```python
from build123d import *

# Parameters (mm, degrees)
F1_DEPTH = 5
F3_DEPTH = 12
F4_R     = 1


# Not quite as in the source:
# - a feature names something its author has since deleted; it is built from what else it names


with BuildPart() as f1:
    # F0 (on Front) → F1 (new body)
    with BuildSketch(Plane.XZ):
        Polygon((3.4641016151, 0), (6.9282032303, 6), (3.4641016151, 12), (-3.4641016151, 12), (-6.9282032303, 6), (-3.4641016151, 0), align=None)
    extrude(amount=F1_DEPTH)

    # F2 (on Top) → F3 (join)
    with BuildSketch(Plane.XY):
        with BuildLine():
            ThreePointArc((-9.1206896552, 11.5080742808), (-17.3757316857, 7.2148156887), (-11.5, 0))
            Line((-11.5, 0), (11.5, 0))
            ThreePointArc((11.5, 0), (17.3757316857, 7.2148156887), (9.1206896552, 11.5080742808))
            ThreePointArc((9.1206896552, 11.5080742808), (0, 9.6223590239), (-9.1206896552, 11.5080742808))
        make_face()
    extrude(amount=F3_DEPTH)

    # F4
    f4_edges = [f1.edges().sort_by_distance(p)[0] for p in [
        (7.482051, 0, 12),
        (7.482051, 0, 0),
    ]]
    fillet(f4_edges, radius=F4_R)


solid = f1.part
```
Work out the finished part from the listing and answer in its coordinate system (mm). A direction names the side the tool comes from. Give positions to 0.01 mm unless a question says otherwise; leave off trailing zeros. Order: outer loops, then holes, each group sorted by start corner. A loop starts at its lowest first (then second) coordinate and runs counter-clockwise, first axis right, second up. Notation, with made-up numbers: (-1.75, 15) - (40.25, 15) arc R29 cw to (40.25, 49) - close; hole circle Ø5 at (61.5, 46). An arc over 180 degrees is marked (long way). One line per item, written item: value. Start each with the question number.
1. Consider line 1 (Y direction, x = -11.5, z = 5.5); line 2 (X direction, y = 11.5, z = 3); line 3 (X direction, y = -1.5, z = 4.75). Determine where each line is inside the solid, lowest interval first.
2. Section A-A, the plane x = 0 is taken. Write down the section's boundary in (y, z).
3. Section D-D, the plane z = 7.5 is taken. Write down the section's boundary in (x, y), then the cut area to 3 significant figures.
4. For a pull along X with two mould halves and no side action, classify faces 4 (the face through (0.131, 9.623, 5.93)), 5 (the face through (0, 5, 0)), 6 (the face through (5.22, -2.62, 8.96)) as released by +X, released by -X, zero draft, split by the parting line, or undercut.
5. Section C-C, the plane y = -3.25 is taken. Write down the section's boundary in (x, z), then the cut area to 3 significant figures.
6. Section B-B, the plane z = 5.25 is taken. Write down the section's boundary in (x, y).
7. Each of these flat-tipped pins is pushed along its axis until it touches: pin 1 Ø2 at (x, z) = (-12, 3.5) entering from -Y; pin 2 Ø1 at (y, z) = (-2.5, 1.5) entering from -X; pin 3 Ø1 at (x, z) = (5, 10.5) entering from +Y. Where does it stop, or does it pass through?
8. Which of the six approach directions +Z, -Z, +X, -X, +Y, -Y give full straight-line access (tool end or side, diameter ignored) to faces 1 (the face through (9, 0, 6)), 2 (the face through (-7.426, 0.301, 0.285)), 3 (the face through (7.538, 0.301, 0.285))?
Filled sheet:
1. line 1: 0 to 12
1. line 2: -13.9 to -9.1, 9.1 to 13.9
1. line 3: -6.21 to 6.21
2. outline: (-5, 0) - (8.62, 0) arc R1 ccw to (9.62, 1) - (9.62, 11) arc R1 ccw to (8.62, 12) - (-5, 12) - close
3. outline: (-11.5, 0) - (-6.06, 0) - (-6.06, -5) - (6.06, -5) - (6.06, 0) - (11.5, 0) arc R6 ccw (long way) to (9.12, 11.51) arc R23 cw to (-9.12, 11.51) arc R6 ccw (long way) to start
3. area: 417 mm²
4. face 4: undercut
4. face 5: zero draft
4. face 6: released by +X
5. outline: (-6.93, 6) - (-3.46, 0) - (3.46, 0) - (6.93, 6) - (3.46, 12) - (-3.46, 12) - close
5. area: 125 mm²
6. outline: (-11.5, 0) - (-6.5, 0) - (-6.5, -5) - (6.5, -5) - (6.5, 0) - (11.5, 0) arc R6 ccw (long way) to (9.12, 11.51) arc R23 cw to (-9.12, 11.51) arc R6 ccw (long way) to start
7. pin 1: y = 0
7. pin 2: x = -4.62
7. pin 3: y = 10.29
8. face 1: +X, -Y
8. face 2: -Z, -X, -Y
8. face 3: -Z, +X, -Y
